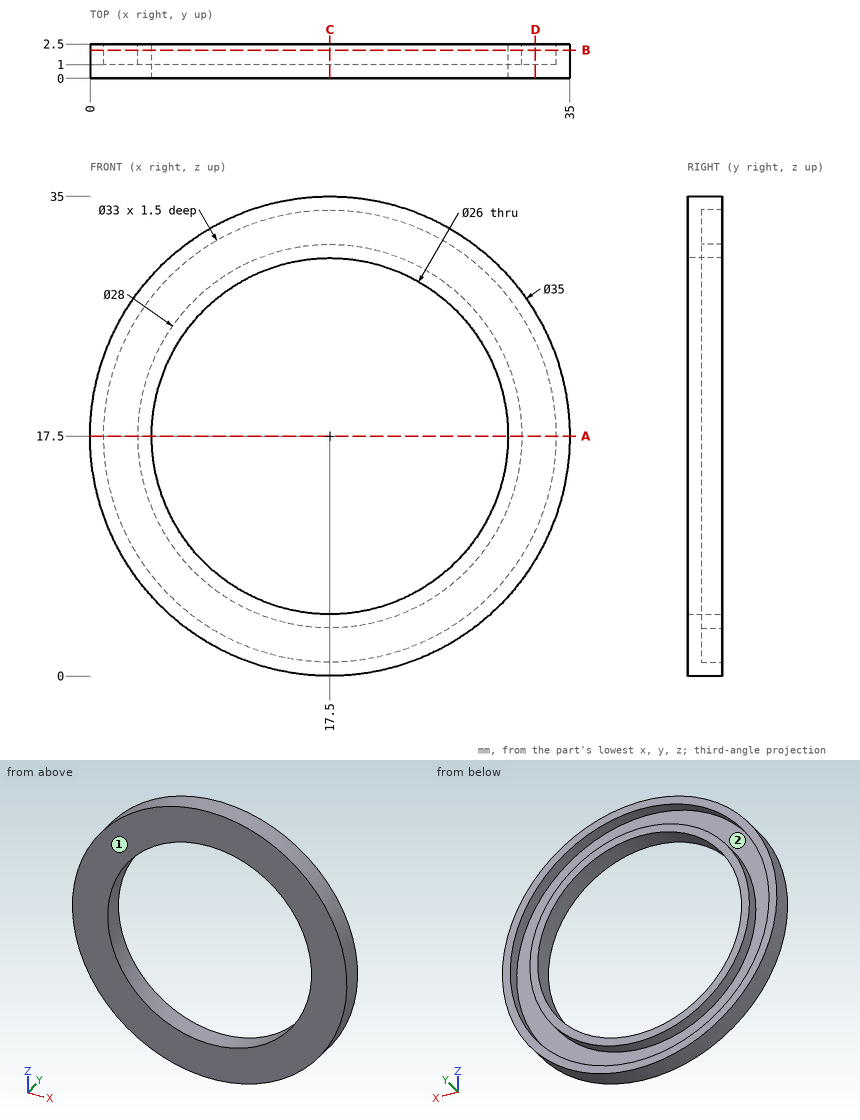
Input: dimensioned drawing with shaded views. Units: mm. Origin: part minimum x, y, z. A direction names the side the tool comes from. Coordinates: 2 decimals unless noted, no trailing zeros. Loops run counter-clockwise (first coordinate to the right, second up) from the corner with the lowest first, then second, coordinate; pieces in that order, holes last. Notation, with made-up numbers: (1.25, -30.75) -> (8.25, -30.75) arc R31 ccw to (8.25, -0.75) -> close; hole circle Ø5 at (-1, 22.5). An arc over 180 degrees is marked (long way). Use a Markdown table: item, result. Add a question column.
(1) Line query: line 1 along X through (y, z) = (1.95, 17.5); line 2 along X through (y, z) = (1.4, 22.5); line 3 along X through (y, z) = (0.4, 18). Output: solid intervals per line, ascending.
(2) Section query C-C, the plane x = 17.5. Return loops of the section in (y, z), plus the area to 3 significant figures.
(3) Access query for the marked faces 1 and 2. Directions: +Z, -Z, +X, -X, +Y, -Y. A direction counts if a zero-diameter tool reaches every point of the face in a straight line with its end or side. Return the directions, or none.
(4) Section query A-A, the plane z = 17.5. Return loops of the section in (x, y), plus the area to 3 significant figures.
(5) Pin query (flat end, axial travel): pin 1 Ø16.5 at (x, z) = (10.5, 18) entering from +Y; pin 2 Ø1.5 at (x, y) = (24.5, 2) entering from +Z. Return the tip coordinate at first contact, or that it passes through.
(6) Section query D-D, the plane x = 32.5. Return loops of the section in (y, z).
(7) Section query B-B, the plane y = 2.05. Return loops of the section in (x, z).
Answer:
| question | item | result |
|---|---|---|
| 1 | line 1 | x = 0 to 1, 3.5 to 4.5, 30.5 to 31.5, 34 to 35 |
| 1 | line 2 | x = 0.73 to 1.78, 4.42 to 5.5, 29.5 to 30.58, 33.22 to 34.27 |
| 1 | line 3 | x = 0.01 to 4.51, 30.49 to 34.99 |
| 2 | outline | (0, 0) -> (2.5, 0) -> (2.5, 1) -> (1, 1) -> (1, 3.5) -> (2.5, 3.5) -> (2.5, 4.5) -> (0, 4.5) -> close; (0, 30.5) -> (2.5, 30.5) -> (2.5, 31.5) -> (1, 31.5) -> (1, 34) -> (2.5, 34) -> (2.5, 35) -> (0, 35) -> close |
| 2 | area | 15.0 mm^2 |
| 3 | face 1 | +Z, -Z, +X, -X, -Y |
| 3 | face 2 | +Y |
| 4 | outline | (0, 0) -> (4.5, 0) -> (4.5, 2.5) -> (3.5, 2.5) -> (3.5, 1) -> (1, 1) -> (1, 2.5) -> (0, 2.5) -> close; (30.5, 0) -> (35, 0) -> (35, 2.5) -> (34, 2.5) -> (34, 1) -> (31.5, 1) -> (31.5, 2.5) -> (30.5, 2.5) -> close |
| 4 | area | 15.0 mm^2 |
| 5 | pin 1 | stops at y = 2.5 |
| 5 | pin 2 | stops at z = 33.85 |
| 6 | outline | (0, 8.49) -> (2.5, 8.49) -> (2.5, 10.63) -> (1, 10.63) -> (1, 24.37) -> (2.5, 24.37) -> (2.5, 26.51) -> (0, 26.51) -> close |
| 7 | outline | circle Ø35 at (17.5, 17.5); circle Ø28 at (17.5, 17.5); hole circle Ø33 at (17.5, 17.5); hole circle Ø26 at (17.5, 17.5) |
